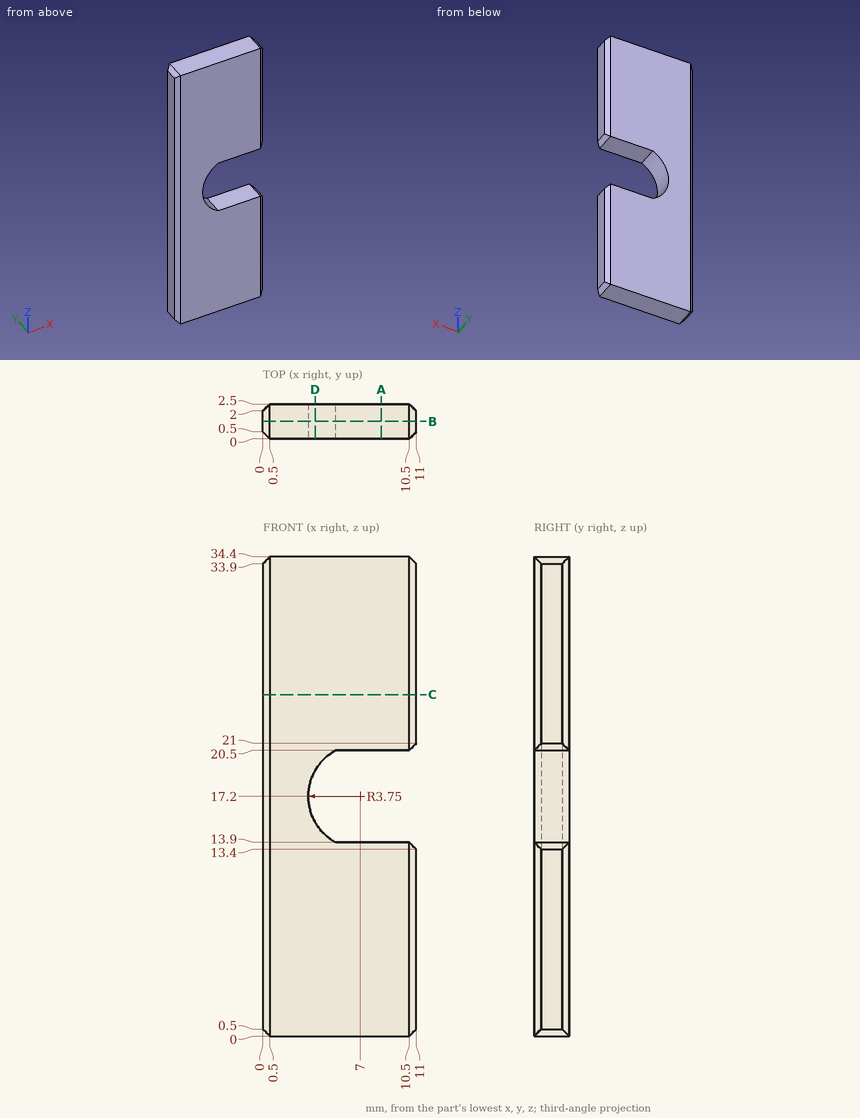
Geometry: see drawing. Coordinates: mm, zero at the bounding-box minimum. Round coordinates to 2 decimals unless told otherwise and drop trailing zeros. Loops run counter-clockwise (first coordinate to the right, second up) from the corner with the lowest first, then second, coordinate; pieces in that order, holes last. Notation, with made-up numbers: (48.25, 1.5) - (64.25, 1.5) arc R17 ccw to (64.25, 27.5) - close; hole circle Ø2 at (6.5, 77.25). An arc over 180 degrees is marked (long way). Write item = value, one per line. Start each with the question number.
(1) Section query D-D, the plane x = 3.75. Output: boundary loops of the cut face in (y, z).
(2) Section query B-B, the plane y = 1.25. Output: boundary loops of the cut face in (x, z).
(3) Section query C-C, the plane z = 24.5. Output: boundary loops of the cut face in (x, y), plus the area to 3 significant figures.
(4) Ray query, line 1 along Z through (x, y) = (10, 0.85); line 2 along Z through (x, y) = (5, 1.3); line 3 along X through (y, z) = (0.45, 17). Return the intervals inside material, ascending. Write a range as from..to.
(5) Pin query (flat end, axial travel): pin 1 (1.2 mm diameter, centred on x = 7, y = 1, fed in from -Z). Return the tip coordinate at first contact, or that it passes through.
(6) Section query A-A, the plane x = 8.5. Output: boundary loops of the cut face in (y, z), plus the area to 3 significant figures.
Conclusion:
q1.outline = (0, 0) - (2.5, 0) - (2.5, 15.33) - (0, 15.33) - close; (0, 19.07) - (2.5, 19.07) - (2.5, 34.4) - (0, 34.4) - close
q2.outline = (0, 0.5) - (0.5, 0) - (10.5, 0) - (11, 0.5) - (11, 13.4) - (10.5, 13.9) - (5.22, 13.9) arc R3.75 cw to (5.22, 20.5) - (10.5, 20.5) - (11, 21) - (11, 33.9) - (10.5, 34.4) - (0.5, 34.4) - (0, 33.9) - close
q3.outline = (0, 0.5) - (0.5, 0) - (10.5, 0) - (11, 0.5) - (11, 2) - (10.5, 2.5) - (0.5, 2.5) - (0, 2) - close
q3.area = 27.0 mm2
q4.line_1 = 0..13.9, 20.5..34.4
q4.line_2 = 0..14.03, 20.37..34.4
q4.line_3 = 0.05..3.26
q5.pin_1 = 0
q6.outline = (0, 0) - (2.5, 0) - (2.5, 13.9) - (0, 13.9) - close; (0, 20.5) - (2.5, 20.5) - (2.5, 34.4) - (0, 34.4) - close
q6.area = 69.5 mm2
